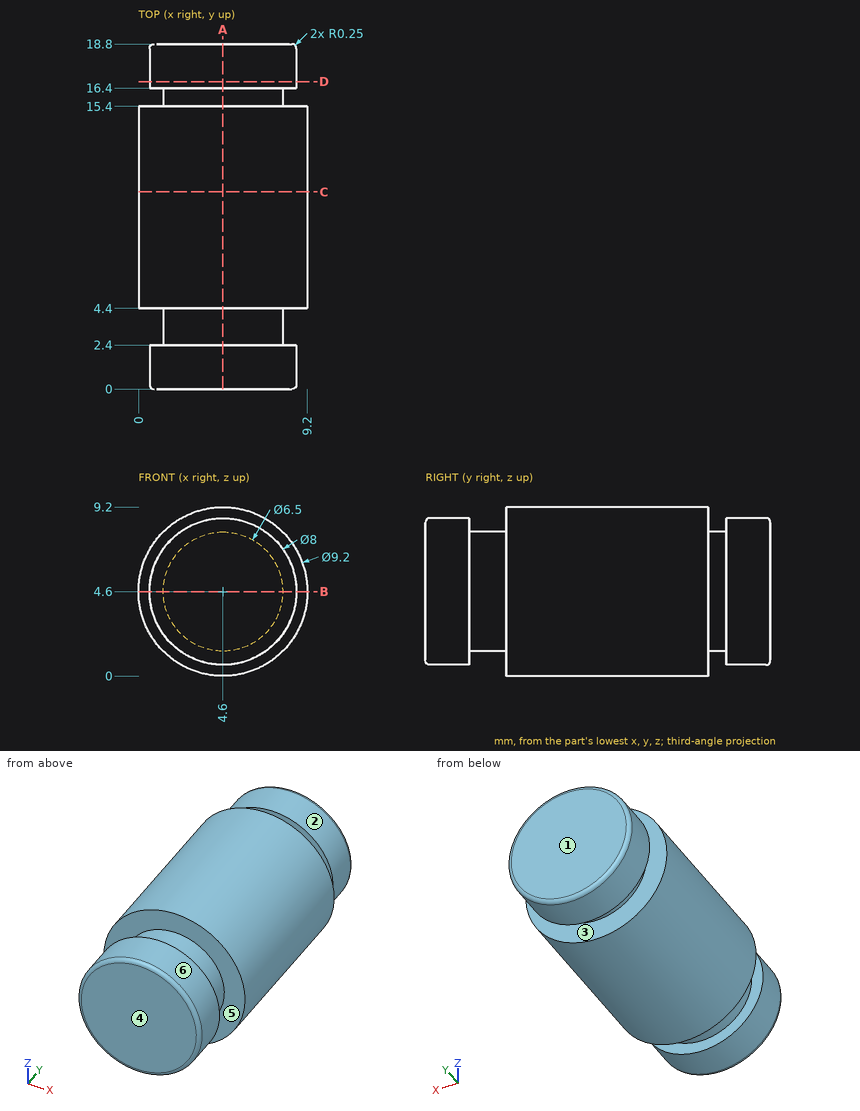
Could you check a few things on this drawing? It's one solid part, dimensions in mm from its lowest x, y, z. A direction names the side the tool comes from. Round coordinates to 2 decimals unless told otherwise and drop trailing zeros. Order: outer loops, then holes, each group sorted by start corner. A loop starts at its lowest first (then second) coordinate and runs counter-clockwise, first axis right, second up.
Q1. Imagine slicing it at C-C, the plane y = 10.75. List the corners of the cut face in (x, z) for me.
Geometry says:
outline: circle Ø9.2 at (4.6, 4.6)
Q2. I'm going to push flat-ended pins straight in: P1, Ø2, axis at y = 8.5, z = 7.5, coming from the -X side; P2, Ø1, axis at y = 10, z = 3, coming from the +X side. Where does each tip first touch, or does it pass through?
Geometry says:
P1: stops at x = 0.41
P2: stops at x = 9.07
Q3. Imagine slicing it at A-A, the plane x = 4.6. List the corners of the cut face in (y, z) for me.
Geometry says:
outline: (0, 0.85) arc R0.25 ccw to (0.25, 0.6) - (2.4, 0.6) - (2.4, 1.35) - (4.4, 1.35) - (4.4, 0) - (15.4, 0) - (15.4, 1.35) - (16.4, 1.35) - (16.4, 0.6) - (18.55, 0.6) arc R0.25 ccw to (18.8, 0.85) - (18.8, 8.35) arc R0.25 ccw to (18.55, 8.6) - (16.4, 8.6) - (16.4, 7.85) - (15.4, 7.85) - (15.4, 9.2) - (4.4, 9.2) - (4.4, 7.85) - (2.4, 7.85) - (2.4, 8.6) - (0.25, 8.6) arc R0.25 ccw to (0, 8.35) - close
Q4. Please list where these lines run through material, in increasing order: probe 1 along Y at (x, z) = (2.25, 0.75); probe 2 along Z at (x, y) = (4.5, 10.75); probe 3 along Z at (x, y) = (5.25, 1.75).
Geometry says:
probe 1: y = 4.4 to 15.4
probe 2: z = 0 to 9.2
probe 3: z = 0.65 to 8.55
Q5. Which directions (+Z, -Z, +X, -X, +Y, -Y) give clear straight access to the entire face, cutting with the end or side of a thin tool? Please do the marked faces 4, 5 and 6.
Geometry says:
face 4: +Z, -Z, +X, -X, -Y
face 5: none
face 6: -Y
Q6. Thinking about a two-plate mould opening in Y: for the marked faces 1, 2 and 3, which applies, released by +Y, released by -Y, zero draft, split by the parting line, or undercut?
Geometry says:
face 1: released by +Y
face 2: zero draft
face 3: undercut
Q7. Imagine slicing it at D-D, the plane y = 16.75. List the corners of the cut face in (x, z) for me, then the cut area to 3 significant figures.
Geometry says:
outline: circle Ø8 at (4.6, 4.6)
area: 50.3 mm2
Q8. Imagine slicing it at B-B, the plane z = 4.6. List the corners of the cut face in (x, y) for me.
Geometry says:
outline: (0, 4.4) - (1.35, 4.4) - (1.35, 2.4) - (0.6, 2.4) - (0.6, 0.25) arc R0.25 ccw to (0.85, 0) - (8.35, 0) arc R0.25 ccw to (8.6, 0.25) - (8.6, 2.4) - (7.85, 2.4) - (7.85, 4.4) - (9.2, 4.4) - (9.2, 15.4) - (7.85, 15.4) - (7.85, 16.4) - (8.6, 16.4) - (8.6, 18.55) arc R0.25 ccw to (8.35, 18.8) - (0.85, 18.8) arc R0.25 ccw to (0.6, 18.55) - (0.6, 16.4) - (1.35, 16.4) - (1.35, 15.4) - (0, 15.4) - close
